The model under review builds one solid part; all positions refer to its coordinate system, in mm. Face numbers are marked on the shaded views. A direction names the side the tool comes from. Give positions to 0.01 mm unless a question says otherwise; leave off trailing zeros. Write item = value, one per line. Start each with the question number.
1. For P1, Ø7.5, axis at x = 10, z = 7, coming from the -Y side; P2, Ø1, axis at x = 7.5, y = 171.5, coming from the +Z side; P3, Ø8, axis at x = 14, y = 151.5, coming from the -Z side; P4, Ø7.5, axis at x = -10.5, z = 11, coming from the -Y side, all flat-tipped, find the tip position at first contact; note any pin that passes through.
2. Machinability: for the marked faces 1 and 2, which of the approach directions +Z, -Z, +X, -X, +Y, -Y give a long, thin tool a straight path to every point of the face, cutting with its end or side? Answer none if there is none.
3. Mouldability with a two-part tool opening along X and no side actions: class the marked faces 3, 4 and 5 as pulls with the +X half, pulls with the -X half, needs draft (parallel to the pull), parting line crosses it, or undercut.
4. Wall thickness on probe 1 along X at (y, z) = (58.5, 19); probe 2 along X at (y, z) = (101, -13.5); probe 3 along Z at (x, y) = (-31.5, 138.5): over which ranges is each line inside the solid? List them lowest first.
5. We need section B-B, the plane z = 18.5. State how many separate pieces and enclosed holes the cut face has, and give its area (3 significant figures).
from build123d import *

# Parameters (mm, degrees)
SKETCH1_R               = 42.350766569
SKETCH1_R_2             = 34.350766569
BOSS_EXTRUDE1_DEPTH     = 250
SKETCH2_R               = 2.5
CUT_EXTRUDE1_DEPTH      = 43.350766569
CUT_EXTRUDE1_DEPTH_BACK = 43.350766569
SKETCH3_R               = 2.5
CUT_EXTRUDE2_DEPTH      = 43.350766669
CUT_EXTRUDE2_DEPTH_BACK = 43.350766669
CUT_EXTRUDE3_DEPTH      = 249.0000001
CIRPATTERN1_COUNT       = 4
SKETCH6_R               = 34.350766569
SKETCH6_R_2             = 12.25
BOSS_EXTRUDE3_DEPTH     = 10
SKETCH8_R               = 12.25
BOSS_EXTRUDE6_DEPTH     = 90
SKETCH9_R               = 34.350766569
SKETCH9_R_2             = 9.75
BOSS_EXTRUDE7_DEPTH     = 10


with BuildPart() as part:
    # Sketch1 → Boss-Extrude1 (new body)
    with BuildSketch(Plane(origin=(0, 0, 0), x_dir=(1, 0, 0), z_dir=(0, 1, 0))):
        Circle(SKETCH1_R)
        Circle(SKETCH1_R_2, mode=Mode.SUBTRACT)
    extrude(amount=BOSS_EXTRUDE1_DEPTH)

    # Sketch2 → Cut-Extrude1 (cut, two sides)
    with BuildSketch(Plane(origin=(0, 0, 0), x_dir=(0, 0, -1), z_dir=(1, 0, 0))) as cut_extrude1_sk:
        with Locations((0, 242.5)):
            Circle(SKETCH2_R)
    extrude(amount=CUT_EXTRUDE1_DEPTH, mode=Mode.SUBTRACT)
    extrude(cut_extrude1_sk.sketch, amount=-CUT_EXTRUDE1_DEPTH_BACK, mode=Mode.SUBTRACT)

    # Sketch3 → Cut-Extrude2 (cut, two sides)
    with BuildSketch(Plane.XY) as cut_extrude2_sk:
        with Locations((0, 242.5)):
            Circle(SKETCH3_R)
    extrude(amount=CUT_EXTRUDE2_DEPTH, mode=Mode.SUBTRACT)
    extrude(cut_extrude2_sk.sketch, amount=-CUT_EXTRUDE2_DEPTH_BACK, mode=Mode.SUBTRACT)

    # Sketch4 → Cut-Extrude3 (cut, through all)
    with BuildSketch(Plane(origin=(0, 2, 0), x_dir=(1, 0, 0), z_dir=(0, 1, 0))):
        with BuildLine():
            Line((31.007174401, 23.936106589), (23.936106589, 31.007174401))
            Line((23.936106589, 31.007174401), (25.350320151, 32.421387963))
            Line((25.350320151, 32.421387963), (26.410980323, 31.360727791))
            Line((26.410980323, 31.360727791), (27.369199622, 32.31894709))
            ThreePointArc((27.369199622, 32.31894709), (29.946514229, 29.946514229), (32.31894709, 27.369199622))
            Line((32.31894709, 27.369199622), (31.360727791, 26.410980323))
            Line((31.360727791, 26.410980323), (32.421387963, 25.350320151))
            Line((32.421387963, 25.350320151), (31.007174401, 23.936106589))
        make_face()
    cut_extrude3 = extrude(amount=CUT_EXTRUDE3_DEPTH, mode=Mode.SUBTRACT)

    # CirPattern1: Cut-Extrude3 ×4 about axis
    cirpattern1_axis = Axis((0, 0, 0), (0, 1, 0))
    for i in range(1, CIRPATTERN1_COUNT):
        add(cut_extrude3.rotate(cirpattern1_axis, i * 360 / CIRPATTERN1_COUNT), mode=Mode.SUBTRACT)

    # Sketch6 → Boss-Extrude3 (add)
    with BuildSketch(Plane(origin=(0, 0, 0), x_dir=(1, 0, 0), z_dir=(0, 1, 0))):
        Circle(SKETCH6_R)
        with Locations((-13.281800184, 13.281800184)):
            Circle(SKETCH6_R_2, mode=Mode.SUBTRACT)
        with Locations((13.281800184, 13.281800184)):
            Circle(SKETCH6_R_2, mode=Mode.SUBTRACT)
        with Locations((13.281800184, -13.281800184)):
            Circle(SKETCH6_R_2, mode=Mode.SUBTRACT)
        with Locations((-13.281800184, -13.281800184)):
            Circle(SKETCH6_R_2, mode=Mode.SUBTRACT)
    extrude(amount=BOSS_EXTRUDE3_DEPTH)

    # Sketch8 → Boss-Extrude6 (add)
    with BuildSketch(Plane(origin=(0, 10, 0), x_dir=(1, 0, 0), z_dir=(0, 1, 0))):
        with BuildLine():
            ThreePointArc((0, 13.281800184), (-22.67345116, 22.67345116), (-13.281800184, 0))
            ThreePointArc((-13.281800184, 0), (-22.67345116, -22.67345116), (0, -13.281800184))
            ThreePointArc((0, -13.281800184), (22.67345116, -22.67345116), (13.281800184, 0))
            ThreePointArc((13.281800184, 0), (22.67345116, 22.67345116), (0, 13.281800184))
        make_face()
        with Locations((-13.281800184, -13.281800184)):
            Circle(SKETCH8_R, mode=Mode.SUBTRACT)
        with Locations((13.281800184, -13.281800184)):
            Circle(SKETCH8_R, mode=Mode.SUBTRACT)
        with Locations((13.281800184, 13.281800184)):
            Circle(SKETCH8_R, mode=Mode.SUBTRACT)
        with Locations((-13.281800184, 13.281800184)):
            Circle(SKETCH8_R, mode=Mode.SUBTRACT)
    extrude(amount=BOSS_EXTRUDE6_DEPTH)

    # Sketch9 → Boss-Extrude7 (add)
    with BuildSketch(Plane(origin=(0, 100, 0), x_dir=(1, 0, 0), z_dir=(0, 1, 0))):
        Circle(SKETCH9_R)
        with Locations((-13.281800184, 13.281800184)):
            Circle(SKETCH9_R_2, mode=Mode.SUBTRACT)
        with Locations((13.281800184, 13.281800184)):
            Circle(SKETCH9_R_2, mode=Mode.SUBTRACT)
        with Locations((13.281800184, -13.281800184)):
            Circle(SKETCH9_R_2, mode=Mode.SUBTRACT)
        with Locations((-13.281800184, -13.281800184)):
            Circle(SKETCH9_R_2, mode=Mode.SUBTRACT)
    extrude(amount=BOSS_EXTRUDE7_DEPTH)


solid = part.part
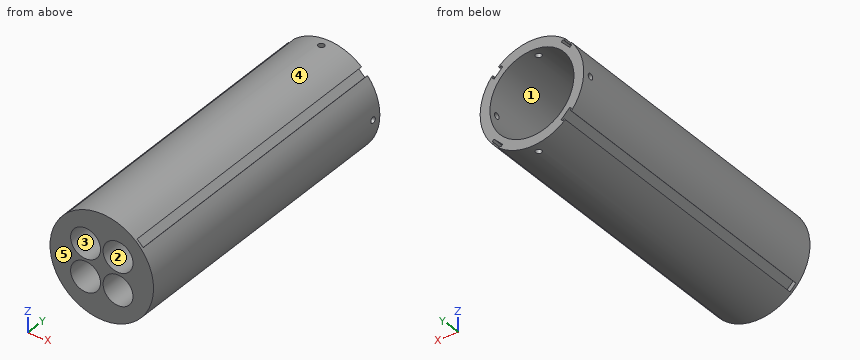
Model answer:
q1.P1 = 100
q1.P2 = 41.77
q1.P3 = -41.15
q1.P4 = through
q2.face_1 = +Y
q2.face_2 = -Y
q3.face_3 = undercut
q3.face_4 = parting line crosses it
q3.face_5 = needs draft
q4.probe_1 = -37.85 to -28.62, -25.27 to -24.12, -2.45 to -1.29, 1.29 to 2.45, 24.12 to 25.27, 28.62 to 37.85
q4.probe_2 = -40.14 to -23.03, -3.53 to 3.53, 23.03 to 40.14
q4.probe_3 = -26.55 to -26.27, -24.43 to -13.7, 13.7 to 24.43, 26.27 to 26.55
q5.separate_pieces = 3
q5.enclosed_holes = 3
q5.area = 5,370 mm2
